from build123d import *

# Parameters (mm, degrees)
F0_W      = 60
F0_H      = 15
F1_DEPTH  = 5
F2_W      = 60
F2_H      = 5
F3_DEPTH  = 10
F5_DEPTH  = 2.5
F6_R      = 1.75
F7_DEPTH  = 2.5
F9_DEPTH  = 2.5
F10_R     = 1.75
F11_DEPTH = 2.5
F12_W     = 64
F12_H     = 19
F12_W_2   = 60
F12_H_2   = 15
F13_DEPTH = 0.2


with BuildPart() as f1:
    # F0 (on Top) → F1 (new body)
    with BuildSketch(Plane.XY):
        with Locations((30, 7.5)):
            Rectangle(F0_W, F0_H)
    extrude(amount=F1_DEPTH)

    # F2 (on face) → F3 (join)
    with BuildSketch(Plane.XY.offset(5)):
        with Locations((30, 2.5)):
            Rectangle(F2_W, F2_H)
    extrude(amount=F3_DEPTH)

    # F4 (on face) → F5 (cut)
    with BuildSketch(Plane.XY.offset(5)):
        Polygon((8.290897, 10), (6.645448, 12.85), (3.354552, 12.85), (1.709103, 10), (3.354552, 7.15), (6.645448, 7.15), align=None)
        Polygon((18.348632, 10), (16.674316, 12.9), (13.325684, 12.9), (11.651368, 10), (13.325684, 7.1), (16.674316, 7.1), align=None)
        Polygon((28.406367, 10), (26.703183, 12.95), (23.296817, 12.95), (21.593633, 10), (23.296817, 7.05), (26.703183, 7.05), align=None)
        Polygon((38.464102, 10), (36.732051, 13), (33.267949, 13), (31.535898, 10), (33.267949, 7), (36.732051, 7), align=None)
        Polygon((46.760918, 13.05), (43.239082, 13.05), (41.478163, 10), (43.239082, 6.95), (46.760918, 6.95), (48.521837, 10), align=None)
        Polygon((58.579572, 10), (56.789786, 13.1), (53.210214, 13.1), (51.420428, 10), (53.210214, 6.9), (56.789786, 6.9), align=None)
    extrude(amount=-F5_DEPTH, mode=Mode.SUBTRACT)

    # F6 (on face) → F7 (cut, through all)
    with BuildSketch(Plane.XY.offset(2.5)):
        with Locations((5, 10)):
            Circle(F6_R)
        with Locations((15, 10)):
            Circle(F6_R)
        with Locations((25, 10)):
            Circle(F6_R)
        with Locations((35, 10)):
            Circle(F6_R)
        with Locations((45, 10)):
            Circle(F6_R)
        with Locations((55, 10)):
            Circle(F6_R)
    extrude(amount=-F7_DEPTH, mode=Mode.SUBTRACT)

    # F8 (on face) → F9 (cut)
    with BuildSketch(Plane(origin=(0, 5, 0), x_dir=(-1, 0, 0), z_dir=(0, 1, 0))):
        Polygon((-51.420428, 10), (-53.210214, 13.1), (-56.789786, 13.1), (-58.579572, 10), (-56.789786, 6.9), (-53.210214, 6.9), align=None)
        Polygon((-43.239082, 13.05), (-46.760918, 13.05), (-48.521837, 10), (-46.760918, 6.95), (-43.239082, 6.95), (-41.478163, 10), align=None)
        Polygon((-33.267949, 13), (-36.732051, 13), (-38.464102, 10), (-36.732051, 7), (-33.267949, 7), (-31.535898, 10), align=None)
        Polygon((-23.296817, 12.95), (-26.703183, 12.95), (-28.406367, 10), (-26.703183, 7.05), (-23.296817, 7.05), (-21.593633, 10), align=None)
        Polygon((-13.325684, 12.9), (-16.674316, 12.9), (-18.348632, 10), (-16.674316, 7.1), (-13.325684, 7.1), (-11.651368, 10), align=None)
        Polygon((-1.709103, 10), (-3.354552, 12.85), (-6.645448, 12.85), (-8.290897, 10), (-6.645448, 7.15), (-3.354552, 7.15), align=None)
    extrude(amount=-F9_DEPTH, mode=Mode.SUBTRACT)

    # F10 (on face) → F11 (cut, through all)
    with BuildSketch(Plane(origin=(0, 2.5, 0), x_dir=(-1, 0, 0), z_dir=(0, 1, 0))):
        with Locations((-55, 10)):
            Circle(F10_R)
        with Locations((-45, 10)):
            Circle(F10_R)
        with Locations((-35, 10)):
            Circle(F10_R)
        with Locations((-25, 10)):
            Circle(F10_R)
        with Locations((-15, 10)):
            Circle(F10_R)
        with Locations((-5, 10)):
            Circle(F10_R)
    extrude(amount=-F11_DEPTH, mode=Mode.SUBTRACT)

    # F12 (on Top) → F13 (join)
    with BuildSketch(Plane.XY):
        with Locations((30, 7.5)):
            Rectangle(F12_W, F12_H)
        with Locations((30, 7.5)):
            Rectangle(F12_W_2, F12_H_2, mode=Mode.SUBTRACT)
    extrude(amount=F13_DEPTH)


solid = f1.part
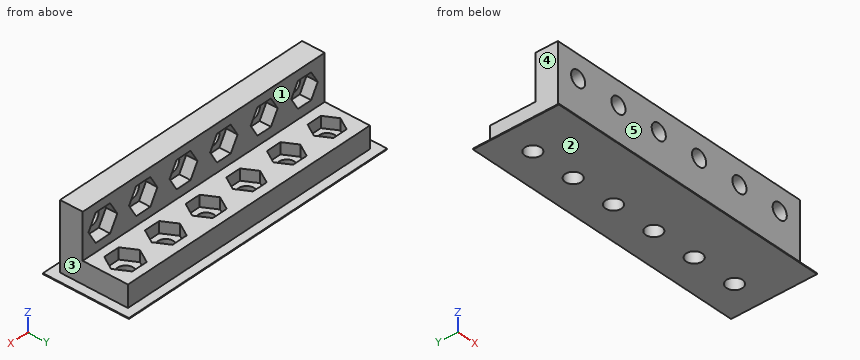
Source: CAD feature listing. Evaluate the final solid. Frame: model axes, mm. Face numbers are marked on the shaded views. A direction names the side the tool comes from. Give positions to 0.01 mm unless a question says otherwise; leave off trailing zeros. Write each loop counter-clockwise with the first axis right and the second up, starting at its lowest first coordinate (ties: lowest second). Pieces come first, ordered by that corner, then holes. Notation, with made-up numbers: (38, 3.5) -> (66, 3.5) arc R17 cw to (66, 35.5) -> close; hole circle Ø11 at (-25, 49.5). An arc over 180 degrees is marked (long way). Return JSON: item names as keys, results as strings. Group by question number.
1. Material intervals for line 1 (Y direction, x = 5, z = 1.6); line 2 (Z direction, x = 16, y = 3.5), sorted ascending. Write a range as from..to.
2. Access query for the marked faces 1 and 2. Directions: +Z, -Z, +X, -X, +Y, -Y. A direction counts if a zero-diameter tool reaches every point of the face in a straight line with its end or side. Return the directions, or none.
3. Section A-A, the plane x = 5. Output: boundary loops of the cut face in (y, z).
4. Section B-B, the plane z = 1.75. Output: boundary loops of the cut face in (x, y), then the cut area to 3 significant figures.
5. Pin query (flat end, axial travel): pin 1 Ø5 at (x, y) = (34.5, 11) entering from +Z; pin 2 Ø3 at (x, z) = (15, 9.5) entering from +Y; pin 3 Ø4 at (x, z) = (54.5, 5) entering from +Y; pin 4 Ø3 at (x, z) = (5, 10) entering from -Y. Return the tip coordinate at first contact, or that it passes through.
6. Section C-C, the plane x = 45. Output: boundary loops of the cut face in (y, z), then the cut area to 3 significant figures.
7. Mould query, pull axis X, two halves, no side actions, for the marked faces 3, 4 and 5. Classes: +X half, -X half, draft (parallel to the pull), parting line (faces both ways), or undercut.
Determined:
{
 "1": {"line 1": "y = 0..8.25, 11.75..15", "line 2": "z = 0..7.1, 12.9..15"},
 "2": {"face 1": "+Z, +X, -X, +Y", "face 2": "-Z, +X, -X, +Y, -Y"},
 "3": {"outline": "(-2, 0) -> (8.25, 0) -> (8.25, 2.5) -> (7.15, 2.5) -> (7.15, 5) -> (5, 5) -> (5, 7.15) -> (2.5, 7.15) -> (2.5, 8.25) -> (0, 8.25) -> (0, 0.2) -> (-2, 0.2) -> close; (0, 11.75) -> (2.5, 11.75) -> (2.5, 12.85) -> (5, 12.85) -> (5, 15) -> (0, 15) -> close; (11.75, 0) -> (17, 0) -> (17, 0.2) -> (15, 0.2) -> (15, 5) -> (12.85, 5) -> (12.85, 2.5) -> (11.75, 2.5) -> close"},
 "4": {"outline": "(0, 0) -> (60, 0) -> (60, 15) -> (0, 15) -> close; hole circle Ø3.5 at (5, 10); hole circle Ø3.5 at (15, 10); hole circle Ø3.5 at (25, 10); hole circle Ø3.5 at (35, 10); hole circle Ø3.5 at (45, 10); hole circle Ø3.5 at (55, 10)", "area": "842 mm2"},
 "5": {"pin 1": "stops at z = 5", "pin 2": "stops at y = 2.5", "pin 3": "stops at y = 15", "pin 4": "passes through"},
 "6": {"outline": "(-2, 0) -> (8.25, 0) -> (8.25, 2.5) -> (6.95, 2.5) -> (6.95, 5) -> (5, 5) -> (5, 6.95) -> (2.5, 6.95) -> (2.5, 8.25) -> (0, 8.25) -> (0, 0.2) -> (-2, 0.2) -> close; (0, 11.75) -> (2.5, 11.75) -> (2.5, 13.05) -> (5, 13.05) -> (5, 15) -> (0, 15) -> close; (11.75, 0) -> (17, 0) -> (17, 0.2) -> (15, 0.2) -> (15, 5) -> (13.05, 5) -> (13.05, 2.5) -> (11.75, 2.5) -> close", "area": "77.8 mm2"},
 "7": {"face 3": "+X half", "face 4": "-X half", "face 5": "draft"}
}
